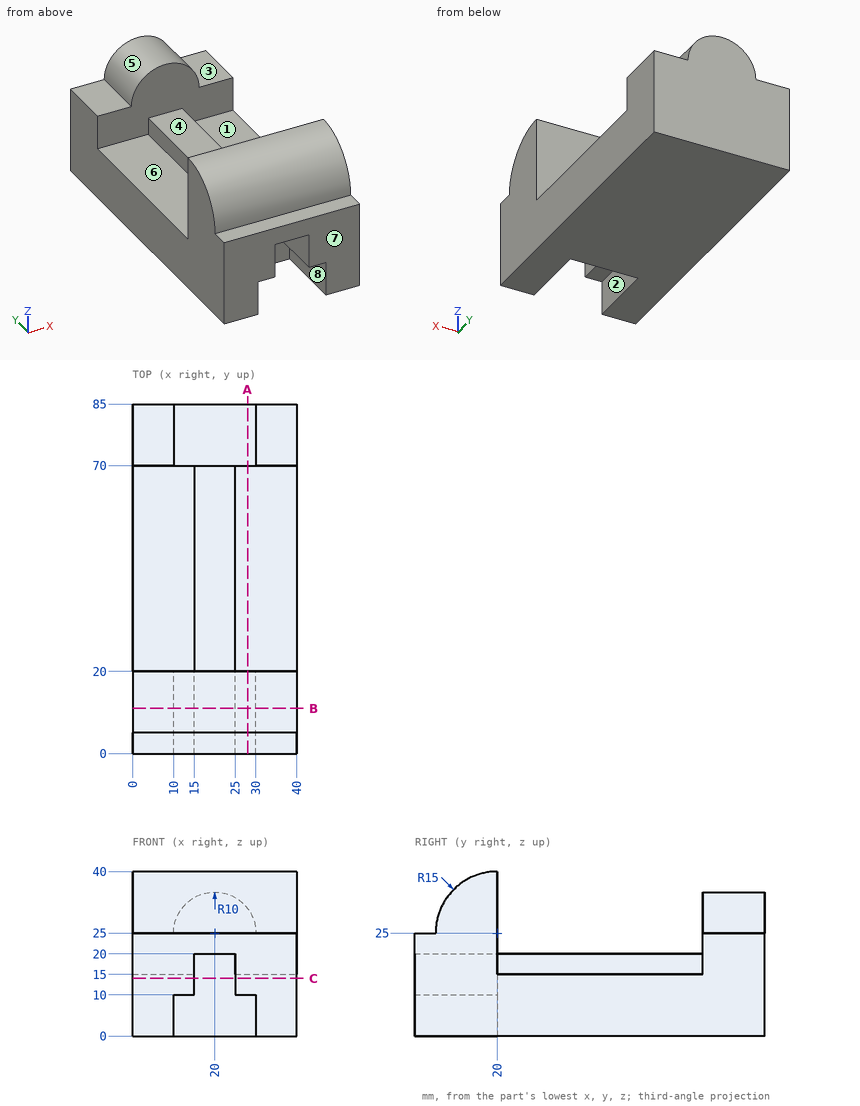
Geometry: see drawing. Coordinates: mm, zero at the bounding-box minimum. A direction names the side the tool comes from. Give positions to 0.01 mm unless a question says otherwise; leave off trailing zeros. Order: outer loops, then holes, each group sorted by start corner. A loop starts at its lowest first (then second) coordinate and runs counter-clockwise, first axis right, second up. Notation, with made-up numbers: (10.5, 63.25) - (48.5, 63.25) arc R14 cw to (48.5, 72.25) - close; hole circle Ø10 at (14, 48.25). An arc over 180 degrees is marked (long way). Use a Markdown table: item, result.
(1) Pin query (flat end, axial travel): pin 1 (4 mm diameter, centred on x = 32, y = 9, fed in from +Z); pin 2 (6 mm diameter, centred on y = 30.5, z = 8, fed in from -X); pin 3 (16.5 mm diameter, centred on x = 4, y = 47.5, fed in from +Z); pin 4 (3 mm diameter, centred on x = 3, y = 74, fed in from +Z). Return the tip coordinate at first contact, or that it passes through.
Computed values:
| item | result |
|---|---|
| pin 1 | stops at z = 37 |
| pin 2 | stops at x = 0 |
| pin 3 | stops at z = 15 |
| pin 4 | stops at z = 25 |
(2) Draft query along Y for the marked faces 6, 7 and 8. Return one class per face: released by +Y, released by -Y, zero draft, split by the parting line, or undercut.
Computed values:
| item | result |
|---|---|
| face 6 | undercut |
| face 7 | released by -Y |
| face 8 | zero draft |
(3) Line query: line 1 (X direction, y = 5.5, z = 18); line 2 (Y direction, x = 2.5, z = 16); line 3 (X direction, y = 14, z = 4). Output: solid intervals per line, ascending. Write a range as from..to.
Computed values:
| item | result |
|---|---|
| line 1 | x = 0..15, 25..40 |
| line 2 | y = 0..20, 70..85 |
| line 3 | x = 0..10, 30..40 |
(4) Section query A-A (x = 28). Output: boundary loops of the cut face in (y, z), then the cut area to 3 significant figures.
Computed values:
| item | result |
|---|---|
| outline | (0, 10) - (20, 10) - (20, 0) - (85, 0) - (85, 31) - (70, 31) - (70, 15) - (20, 15) - (20, 40) arc R15 ccw to (5, 25) - (0, 25) - close |
| area | 1,690 mm2 |
(5) Section query C-C (z = 14). Output: boundary loops of the cut face in (x, y).
Computed values:
| item | result |
|---|---|
| outline | (0, 0) - (15, 0) - (15, 20) - (25, 20) - (25, 0) - (40, 0) - (40, 85) - (0, 85) - close |
(6) Section query B-B (y = 11). Output: boundary loops of the cut face in (x, z), then the cut area to 3 significant figures.
Computed values:
| item | result |
|---|---|
| outline | (0, 0) - (10, 0) - (10, 10) - (15, 10) - (15, 20) - (25, 20) - (25, 10) - (30, 10) - (30, 0) - (40, 0) - (40, 37) - (0, 37) - close |
| area | 1,180 mm2 |
(7) Access query for the marked faces 1, 2, 3, 4 and 5. Directions: +Z, -Z, +X, -X, +Y, -Y. A direction counts if a zero-diameter tool reaches every point of the face in a straight line with its end or side. Return the directions, or none.
Computed values:
| item | result |
|---|---|
| face 1 | +Z, +X |
| face 2 | -Z, -Y |
| face 3 | +Z, +X, +Y |
| face 4 | +Z, +X, -X |
| face 5 | +Z, +Y |
